Work out the finished part from the listing and answer in its coordinate system (mm). Give positions to 0.01 mm unless a question says otherwise; leave off trailing zeros. Order: outer loops, then holes, each group sorted by start corner. A loop starts at its lowest first (then second) coordinate and runs counter-clockwise, first axis right, second up. Notation, with made-up numbers: (82.5, -2.75) -> (128.5, -2.75) arc R17 ccw to (128.5, 3.25) -> close; hole circle Ø2 at (30.5, 76.5). An arc over 180 degrees is marked (long way). Use a Markdown table: item, result. Add a question column.
```python
from build123d import *

# Parameters (mm, degrees)
F0_R     = 37
F0_R_2   = 6.41
F1_DEPTH = 2
F3_DEPTH = 2
F4_R     = 3
F5_DEPTH = 2.001
F6_SIZE2 = 1.6
F6_SIZE  = 1.6


with BuildPart() as f1:
    # F0 (on Front) → F1 (new body)
    with BuildSketch(Plane.XZ):
        Circle(F0_R)
        Circle(F0_R_2, mode=Mode.SUBTRACT)
    extrude(amount=-F1_DEPTH)

    # F2 (on face) → F3 (join)
    with BuildSketch(Plane.XZ):
        with BuildLine():
            Line((12.5, 117), (-12.5, 117))
            Line((-12.5, 117), (-12.5, 34.82456))
            ThreePointArc((-12.5, 34.82456), (0, 37), (12.5, 34.82456))
            Line((12.5, 34.82456), (12.5, 117))
        make_face()
    extrude(amount=-F3_DEPTH)

    # F4 (on face) → F5 (cut, through all)
    with BuildSketch(Plane.XZ):
        with Locations((0, 102)):
            Circle(F4_R)
    extrude(amount=-F5_DEPTH, mode=Mode.SUBTRACT)

    # F6
    f6_edges = [f1.edges().sort_by_distance(p)[0] for p in [
        (-6.41, 2, 0),
    ]]
    chamfer(f6_edges, length=F6_SIZE, length2=F6_SIZE2)


solid = f1.part
```
1) The part is cut by section C-C, the plane y = 1.5. Determine the outline of the cut face in (x, z).
2) The part is cut by section D-D, the plane z = 0. Determine the outline of the cut face in (x, y).
3) Straight lines are drawn through the part: line 1 (Z direction, x = 0, y = 0.15); line 2 (Z direction, x = 0, y = 1.25); line 3 (X direction, y = 0.75, z = 67). For each, find the intervals that lie inside material, in ascending order.
4) Flat-ended cylindrical pins translate along their axes: pin 1 (1 mm diameter, centred on y = 1, z = 94, fed in from -X); pin 2 (7.5 mm diameter, centred on x = 0, z = 0, fed in from +Y); pin 3 (0.6 mm diameter, centred on y = 1, z = 69, fed in from +X). Find the tip coordinate at first contact, or state that the pin passes through.
5) The part is cut by section B-B, the plane x = 0. Determine the outline of the cut face in (y, z), then the cut area to 3 significant figures.
6) Determine the mould class of faces 1 (the cylindrical face through (-0.65, 0.99, 99.07)), 2 (the cylindrical face through (-1.45, 0.99, -36.97)), 3 (the flat face through (-1, 2, 24)) for opening direction X: released by +X, released by -X, zero draft, split by the parting line, or undercut.
7) The part is cut by section A-A, the plane z = 102. Determine the outline of the cut face in (x, y).
A:
| question | item | result |
|---|---|---|
| 1 | outline | (-12.5, 34.82) arc R37 ccw (long way) to (12.5, 34.82) -> (12.5, 117) -> (-12.5, 117) -> close; hole circle Ø15.02 at (0, 0); hole circle Ø6 at (0, 102) |
| 2 | outline | (-37, 0) -> (-6.41, 0) -> (-6.41, 0.4) -> (-8.01, 2) -> (-37, 2) -> close; (6.41, 0) -> (37, 0) -> (37, 2) -> (8.01, 2) -> (6.41, 0.4) -> close |
| 3 | line 1 | -37 to -6.41, 6.41 to 99, 105 to 117 |
| 3 | line 2 | -37 to -7.26, 7.26 to 99, 105 to 117 |
| 3 | line 3 | -12.5 to 12.5 |
| 4 | pin 1 | x = -12.5 |
| 4 | pin 2 | through |
| 4 | pin 3 | x = 12.5 |
| 5 | outline | (0, -37) -> (2, -37) -> (2, -8.01) -> (0.4, -6.41) -> (0, -6.41) -> close; (0, 6.41) -> (0.4, 6.41) -> (2, 8.01) -> (2, 99) -> (0, 99) -> close; (0, 105) -> (2, 105) -> (2, 117) -> (0, 117) -> close |
| 5 | area | 268 mm^2 |
| 6 | face 1 | undercut |
| 6 | face 2 | split by the parting line |
| 6 | face 3 | zero draft |
| 7 | outline | (-12.5, 0) -> (-3, 0) -> (-3, 2) -> (-12.5, 2) -> close; (3, 0) -> (12.5, 0) -> (12.5, 2) -> (3, 2) -> close |
